Could you check a few things on this drawing? It's one solid part, dimensions in mm from its lowest x, y, z. Give positions to 0.01 mm unless a question says otherwise; leave off trailing zeros. Loops run counter-clockwise (first coordinate to the right, second up) from the corner with the lowest first, then second, coordinate; pieces in that order, holes last. Notation, with made-up numbers: (16.5, 89) -> (31.5, 89) arc R22 ccw to (31.5, 111) -> close; hole circle Ø6 at (13.5, 66.25). An arc over 180 degrees is marked (long way). Use CSV: the item, a comma, the result in double quotes.
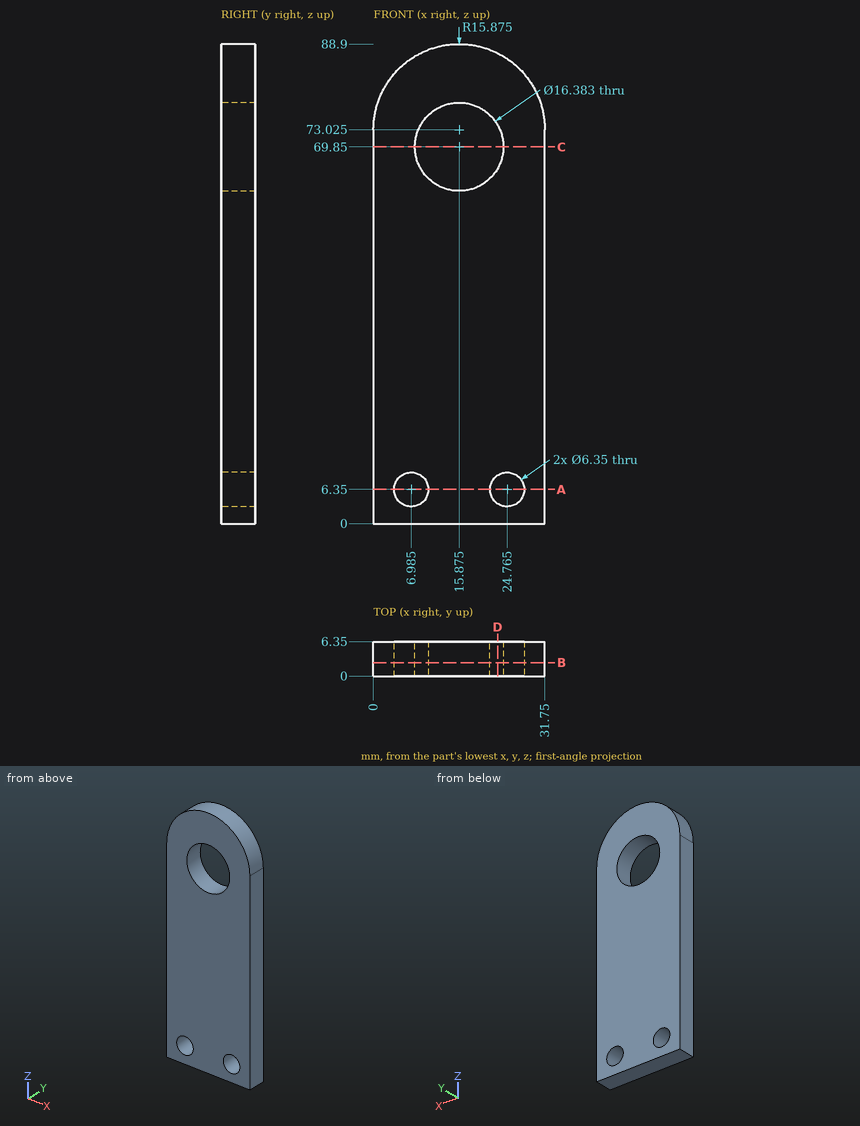
(1) If we section it at D-D, the plane x = 23: Write out the boundary of the cut face in (y, z), then the cut area to 3 significant figures.
Answer sheet:
outline,"(0, 0) -> (6.35, 0) -> (6.35, 3.71) -> (0, 3.71) -> close; (0, 8.99) -> (6.35, 8.99) -> (6.35, 65.81) -> (0, 65.81) -> close; (0, 73.89) -> (6.35, 73.89) -> (6.35, 87.21) -> (0, 87.21) -> close"
area,"469 mm2"
(2) If I drill on L1, parallel to Z at x = 16, y = 2.5; L2, parallel to Z at x = 18.5, y = 5; L3, parallel to X at y = 4, z = 63, over which ranges is the centre line in solid material (lowest first)? Write a range as from..to.
Answer sheet:
L1,"z = 0..61.66, 78.04..88.9"
L2,"z = 0..62.09, 77.61..88.68"
L3,"x = 0..11.38, 20.37..31.75"
(3) If we section it at C-C, the plane z = 69.85: Write out the boundary of the cut face in (x, y).
Answer sheet:
outline,"(0, 0) -> (7.68, 0) -> (7.68, 6.35) -> (0, 6.35) -> close; (24.07, 0) -> (31.75, 0) -> (31.75, 6.35) -> (24.07, 6.35) -> close"
(4) If we section it at A-A, the plane z = 6.35: Write out the boundary of the cut face in (x, y).
Answer sheet:
outline,"(0, 0) -> (3.81, 0) -> (3.81, 6.35) -> (0, 6.35) -> close; (10.16, 0) -> (21.59, 0) -> (21.59, 6.35) -> (10.16, 6.35) -> close; (27.94, 0) -> (31.75, 0) -> (31.75, 6.35) -> (27.94, 6.35) -> close"
(5) If we section it at B-B, the plane y = 2.5: Give the number of separate pieces and of enclosed holes in the cut face, then the cut area to 3 significant figures.
Answer sheet:
separate pieces,"1"
enclosed holes,"3"
area,"2,440 mm2"
